Geometry check sheet. Reference: the model listing, model coordinates, mm. Round coordinates to 2 decimals unless told otherwise and drop trailing zeros. Order: outer loops, then holes, each group sorted by start corner. A loop starts at its lowest first (then second) coordinate and runs counter-clockwise, first axis right, second up. Notation, with made-up numbers: (42, 44) -> (84, 44) arc R19 cw to (84, 57) -> close; hole circle Ø3 at (68, 58). An arc over 180 degrees is marked (long way). Answer as a JSON object with one key per item and string values. Group by question number.
from build123d import *

# Parameters (mm, degrees)
SKETCH1_R            = 7.9375
SKETCH1_R_2          = 3
BOSS_EXTRUDE1_DEPTH  = 1.5875
M6_CLEARANCE_HOLE1_D = 6.6
CUT_EXTRUDE1_DEPTH   = 30.699405508
FILLET1_R            = 1.5875


with BuildPart() as part:
    # Sketch1 → Boss-Extrude1 (new body)
    # profile 1 of 3: a face of its own
    with BuildSketch(Plane.XY):
        Circle(SKETCH1_R)
        Circle(SKETCH1_R_2, mode=Mode.SUBTRACT)
    # profile 2 of 3: a face of its own
    with BuildSketch(Plane.XY):
        with BuildLine():
            ThreePointArc((7.9375, 0), (0, -7.9375), (-7.9375, 0))
            Line((-7.9375, 0), (-7.9375, -28.575))
            Line((-7.9375, -28.575), (7.9375, -28.575))
            Line((7.9375, -28.575), (7.9375, 0))
        make_face()
    # profile 3 of 3: a face of its own
    with BuildSketch(Plane.XY):
        Circle(SKETCH1_R_2)
    extrude(amount=BOSS_EXTRUDE1_DEPTH)

    # M6 Clearance Hole1 (through all)
    with Locations(Plane.XY.offset(1.5875)):
        with Locations((0, 0)):
            Hole(M6_CLEARANCE_HOLE1_D / 2)

    # Sketch4 → Cut-Extrude1 (cut, through all)
    with BuildSketch(Plane.XY.offset(1.5875)):
        Polygon((7.9375, -28.575), (7.9375, -15.441016157), (2.035744182, -27.468766371), (-7.9375, -11.475212377), (-7.9375, -28.575), align=None)
    extrude(amount=-CUT_EXTRUDE1_DEPTH, mode=Mode.SUBTRACT)

    # Fillet1
    fillet1_edges = [part.edges().sort_by_distance(p)[0] for p in [
        (-7.9375, -11.475212377, 0.79375),
        (2.035744182, -27.468766371, 0.79375),
        (7.9375, -15.441016157, 0.79375),
    ]]
    fillet(fillet1_edges, radius=FILLET1_R)


solid = part.part
Item 1: Sectioned sample at A-A, the plane x = 0. Enter the section's corners in (y, z).
Item 2: Sectioned sample at C-C, the plane x = 2.25. Enter the section's corners in (y, z).
Item 3: Mould release check, pull along X, two halves, no side actions. Record for faces 1 (the cylindrical face through (2.43, 2.23, 0.78)), 2 (the flat face through (0, -9, 0)), 3 (the cylindrical face through (1.974, -25.787, 0.783)): pulls with the +X half, pulls with the -X half, needs draft (parallel to the pull), parting line crosses it, or undercut.
Item 4: Sectioned sample at D-D, the plane y = -23. Enter the section's corners in (x, z), then the cut area to 3 significant figures.
Item 5: Thickness scan on L1, parallel to Y at x = 0, z = 0.65; L2, parallel to Y at x = 1.5, z = 0.95; L3, parallel to Y at x = -5.5, z = 1. Record the ranges inside material, lowest first.
Result:
{
 "1": {"outline": "(-24.2, 0) -> (-3.3, 0) -> (-3.3, 1.59) -> (-24.2, 1.59) -> close; (3.3, 0) -> (7.94, 0) -> (7.94, 1.59) -> (3.3, 1.59) -> close"},
 "2": {"outline": "(-25.74, 0) -> (-2.41, 0) -> (-2.41, 1.59) -> (-25.74, 1.59) -> close; (2.41, 0) -> (7.61, 0) -> (7.61, 1.59) -> (2.41, 1.59) -> close"},
 "3": {"face 1": "undercut", "face 2": "needs draft", "face 3": "parting line crosses it"},
 "4": {"outline": "(-0.75, 0) -> (4.23, 0) -> (4.23, 1.59) -> (-0.75, 1.59) -> close", "area": "7.90 mm2"},
 "5": {"L1": "y = -24.2 to -3.3, 3.3 to 7.94", "L2": "y = -25.75 to -2.94, 2.94 to 7.79", "L3": "y = -15.38 to 5.72"}
}
